```python
from build123d import *

# Parameters (mm, degrees)
BOSS_EXTRUDE1_DEPTH = 80
SKETCH3_R           = 40
BOSS_EXTRUDE2_DEPTH = 40
CUT_EXTRUDE3_START  = -40
CUT_EXTRUDE3_DEPTH  = 40


with BuildPart() as part:
    # Sketch2 → Boss-Extrude1 (new body)
    with BuildSketch(Plane(origin=(0, 0, 0), x_dir=(0, 0, -1), z_dir=(1, 0, 0))):
        with BuildLine():
            Line((-80, -40), (0, -40))
            Line((0, -40), (0, -80))
            ThreePointArc((0, -80), (40, -120), (80, -80))
            Line((80, -80), (80, -40))
            Line((80, -40), (80, 0))
            ThreePointArc((80, 0), (68.284271247, 28.284271247), (40, 40))
            Line((40, 40), (-80, 40))
            Line((-80, 40), (-80, -40))
        make_face()
    extrude(amount=BOSS_EXTRUDE1_DEPTH)

    # Sketch3 → Boss-Extrude2 (add)
    with BuildSketch(Plane.XY.offset(80)):
        with Locations((40, 0)):
            Circle(SKETCH3_R)
    extrude(amount=BOSS_EXTRUDE2_DEPTH)

    # Sketch5 → Cut-Extrude3 (cut)
    with BuildSketch(Plane.XY.offset(80).offset(CUT_EXTRUDE3_START)):
        with BuildLine():
            Line((40, 40), (0, 40))
            Line((0, 40), (0, -8.6e-08))
            ThreePointArc((0, -8.6e-08), (11.715728722, 28.284271217), (40, 40))
        make_face()
        with BuildLine():
            Line((80, 40), (40, 40))
            ThreePointArc((40, 40), (68.284271247, 28.284271247), (80, 0))
            Line((80, 0), (80, 40))
        make_face()
        with BuildLine():
            ThreePointArc((40, -40), (11.715728783, -28.284271278), (0, -8.6e-08))
            Line((0, -8.6e-08), (0, -40))
            Line((0, -40), (40, -40))
        make_face()
        with BuildLine():
            Line((80, -40), (80, 0))
            ThreePointArc((80, 0), (68.284271247, -28.284271247), (40, -40))
            Line((40, -40), (80, -40))
        make_face()
    extrude(amount=CUT_EXTRUDE3_DEPTH, mode=Mode.SUBTRACT)


solid = part.part
```
Check sheet for the modelled part. Datum: model origin and axes. Units: mm. A direction names the side the tool comes from. Give positions to 0.01 mm unless a question says otherwise; leave off trailing zeros. Write each loop counter-clockwise with the first axis right and the second up, starting at its lowest first coordinate (ties: lowest second). Pieces come first, ordered by that corner, then holes. Notation, with made-up numbers: (-9.5, 79) -> (29.5, 79) arc R17 ccw to (29.5, 112) -> close; hole circle Ø11 at (-29.5, 58.25). An arc over 180 degrees is marked (long way). Use CSV: the item, a comma, the result in double quotes. Start each with the question number.
Q1. Cross-section at A-A on x = 35. Enter the section's corners in (y, z), and give its area (3 significant figures).
Q2. Cross-section at D-D on x = 25. Enter the section's corners in (y, z), and give its area (3 significant figures).
Q3. Scan lines: line 1 along Z through (x, y) = (15, -32); line 2 along Z through (x, y) = (76, -44); line 3 along Y through (x, z) = (50.5, 5.5). Record each from-to range of solid material in increasing order.
Q4. Cross-section at C-C on y = -16. Enter the section's corners in (x, z), and give its area (3 significant figures).
Q5. Depth check by flat-ended pin: P1, Ø1, axis at x = 13.5, z = 39, coming from the -Y side; P2, Ø12, axis at x = 52.5, y = -64, coming from the +Z side; P3, Ø12, axis at x = 47, z = -24.5, coming from the -Y side. Enter the tip coordinate at first touch or a pass-through.
Q6. Tool access check on faces 1 (the flat face through (39, -60, 0)), 2 (the flat face through (8, -30, 40)), 3 (the flat face through (8, 30, 40)). Record the directions out of +Z, -Z, +X, -X, +Y, -Y that give a thin tool (end or side, any length) a straight path to the whole face; none if there is none.
Q7. Cross-section at B-B on z = 96.5. Enter the section's corners in (x, y), and give its area (3 significant figures).
Working result:
1,outline,"(-80, -80) -> (0, -80) arc R40 ccw to (40, -40) -> (40, 40) -> (39.69, 40) -> (39.69, 120) -> (-39.69, 120) -> (-39.69, 40) -> (-40, 40) -> (-40, 0) -> (-80, 0) arc R40 ccw to start"
1,area,"21,300 mm^2"
2,outline,"(-80, -80) -> (0, -80) arc R40 ccw to (40, -40) -> (40, 40) -> (37.08, 40) -> (37.08, 120) -> (-37.08, 120) -> (-37.08, 40) -> (-40, 40) -> (-40, 0) -> (-80, 0) arc R40 ccw to start"
2,area,"20,900 mm^2"
3,line 1,"z = -80 to 40"
3,line 2,"z = -80 to 0"
3,line 3,"y = -40 to 40"
4,outline,"(0, -80) -> (80, -80) -> (80, 40) -> (76.66, 40) -> (76.66, 120) -> (3.34, 120) -> (3.34, 40) -> (0, 40) -> close"
4,area,"15,500 mm^2"
5,P1,"stops at y = -40"
5,P2,"stops at z = 0"
5,P3,"stops at y = -118.86"
6,face 1,"+Z, +X, -X, -Y"
6,face 2,"+Z, -X, -Y"
6,face 3,"+Z, -X, +Y"
7,outline,"circle Ø80 at (40, 0)"
7,area,"5,030 mm^2"
